Check sheet for the drawn part. Datum: minimum x, y, z corner. Units: mm. A direction names the side the tool comes from. Round coordinates to 2 decimals unless told otherwise and drop trailing zeros. Write each loop counter-clockwise with the first axis right and the second up, starting at its lowest first coordinate (ties: lowest second). Pieces come first, ordered by that corner, then holes. Notation, with made-up numbers: (23, 10.25) - (38, 10.25) arc R29 cw to (38, 45.25) - close; hole circle Ø1 at (23.5, -21). An arc over 180 degrees is marked (long way). Answer as a JSON object with one key per item and string values.
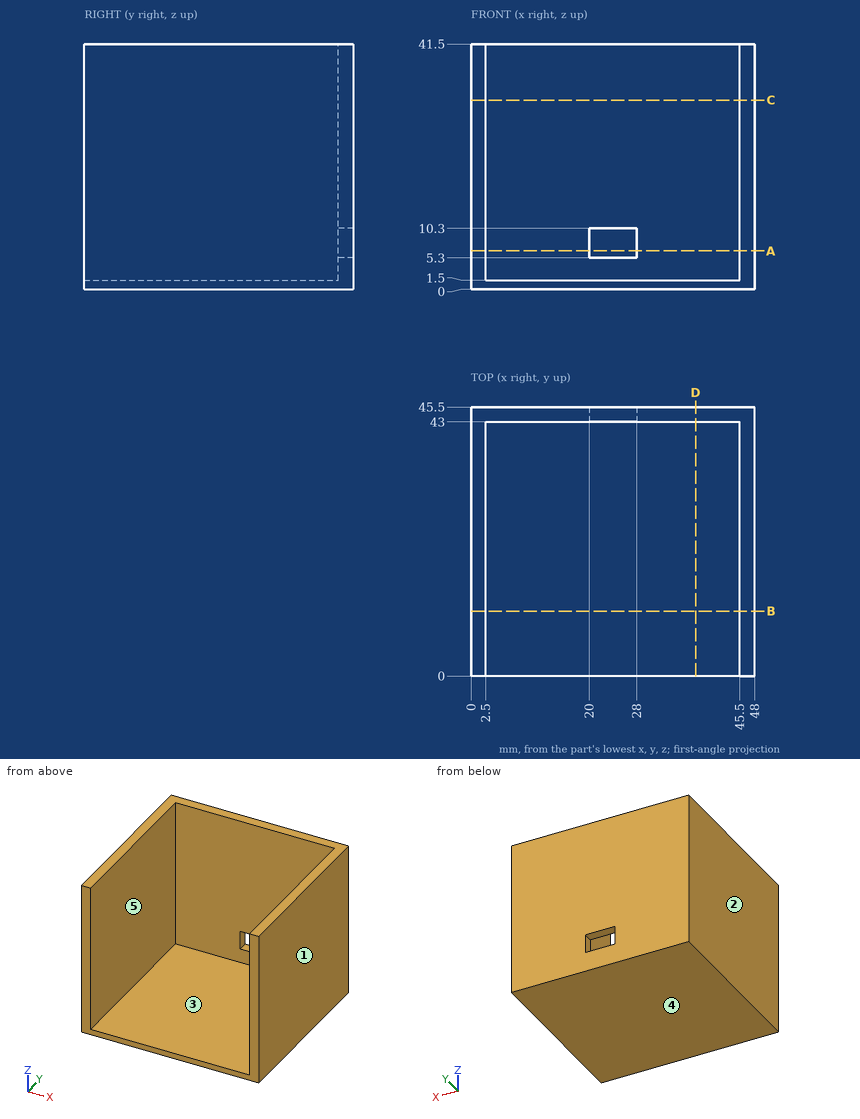
Q1. Section check C-C, the plane z = 32. Record the cut outline in (x, y).
Geometry check:
{"outline": "(0, 0) - (2.5, 0) - (2.5, 43) - (45.5, 43) - (45.5, 0) - (48, 0) - (48, 45.5) - (0, 45.5) - close"}
Q2. Section check A-A, the plane z = 6.5. Record the cut outline in (x, y), then the cut area to 3 significant figures.
Geometry check:
{"outline": "(0, 0) - (2.5, 0) - (2.5, 43) - (20, 43) - (20, 45.5) - (0, 45.5) - close; (28, 43) - (45.5, 43) - (45.5, 0) - (48, 0) - (48, 45.5) - (28, 45.5) - close", "area": "315 mm2"}
Q3. Section check D-D, the plane x = 38. Record the cut outline in (y, z), then the cut area to 3 significant figures.
Geometry check:
{"outline": "(0, 0) - (45.5, 0) - (45.5, 41.5) - (43, 41.5) - (43, 1.5) - (0, 1.5) - close", "area": "168 mm2"}
Q4. Gauge pin test, flat ends, axial feed: P1, Ø0.8, axis at x = 24.5, y = 44.5, coming from the -Z side; P2, Ø13, axis at x = 27, y = 28.5, coming from the +Z side. Record the tip position at first contact, or that the pin passes through.
Geometry check:
{"P1": "stops at z = 0", "P2": "stops at z = 1.5"}
Q5. Section check B-B, the plane y = 11. Record the cut outline in (x, z).
Geometry check:
{"outline": "(0, 0) - (48, 0) - (48, 41.5) - (45.5, 41.5) - (45.5, 1.5) - (2.5, 1.5) - (2.5, 41.5) - (0, 41.5) - close"}
Q6. Release check for a two-part mould opening along X. For the marked faces 1, 2 and 3 record: released by +X, released by -X, zero draft, split by the parting line, or undercut.
Geometry check:
{"face 1": "released by +X", "face 2": "released by -X", "face 3": "undercut"}
Q7. Material ranges on line 1 along X through (y, z) = (39, 4); line 2 along Y through (x, z) = (42, 27); line 3 along Z through (x, y) = (29, 12.5), recorded low to high. Write a range as [from, to].
Geometry check:
{"line 1": "x = [0, 2.5], [45.5, 48]", "line 2": "y = [43, 45.5]", "line 3": "z = [0, 1.5]"}
Q8. Set-up check for the marked faces 4 and 5: record each of +Z, -Z, +X, -X, +Y, -Y from which the full face is reachable in a straight line by a thin tool's end or side.
Geometry check:
{"face 4": "-Z, +X, -X, +Y, -Y", "face 5": "+Z, -Y"}
